Study the drawing (mm; zero at the part's minimum x, y, z) and answer. Coordinates: 2 decimals unless noted, no trailing zeros. Order: outer loops, then holes, each group sorted by start corner. A loop starts at its lowest first (then second) coordinate and runs counter-clockwise, first axis right, second up. Notation, with made-up numbers: (-6, 34) - (14, 34) arc R28 cw to (14, 71) - close; hole circle Ø3 at (49, 63.25). An arc over 180 degrees is marked (long way). Write item = value, one per line.
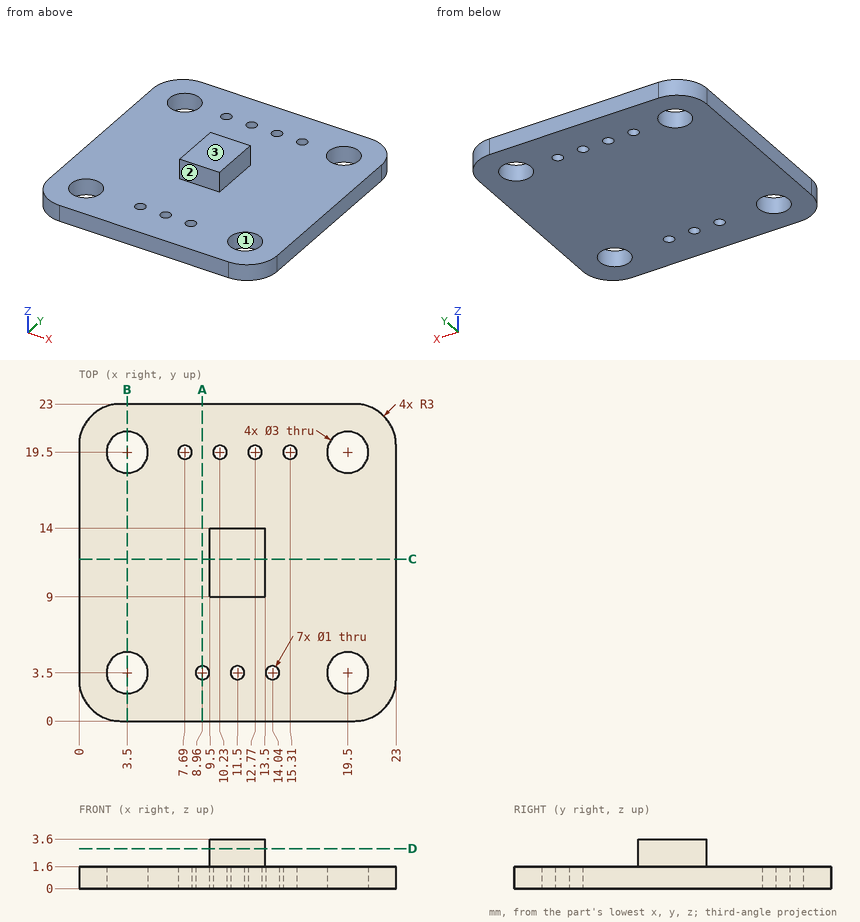
1) Flat-ended cylindrical pins translate along their axes: pin 1 Ø5 at (x, y) = (3.5, 3.5) entering from +Z; pin 2 Ø0.6 at (x, z) = (11, 2.5) entering from +Y; pin 3 Ø2.5 at (x, y) = (3.5, 19.5) entering from -Z; pin 4 Ø2 at (y, z) = (10.5, 3) entering from +X. Find the tip coordinate at first contact, or state that the pin passes through.
Returned:
pin_1 = 1.6
pin_2 = 14
pin_3 = through
pin_4 = 13.5
2) Straight lines are drawn through the part: line 1 along Y through (x, z) = (19.5, 0.9); line 2 along Y through (x, z) = (12.77, 0.6); line 3 along Y through (x, z) = (11.5, 1). For each, find the intervals that lie inside material, in ascending order. Write a range as from..to.
Returned:
line_1 = 0..2, 5..18, 21..23
line_2 = 0..19, 20..23
line_3 = 0..3, 4..23
3) The part is cut by section D-D (z = 2.9). Determine the outline of the cut face in (x, y).
Returned:
outline = (9.5, 9) - (13.5, 9) - (13.5, 14) - (9.5, 14) - close
4) The part is cut by section B-B (x = 3.5). Determine the outline of the cut face in (y, z).
Returned:
outline = (0, 0) - (2, 0) - (2, 1.6) - (0, 1.6) - close; (5, 0) - (18, 0) - (18, 1.6) - (5, 1.6) - close; (21, 0) - (23, 0) - (23, 1.6) - (21, 1.6) - close
5) The part is cut by section A-A (x = 8.96). Determine the outline of the cut face in (y, z).
Returned:
outline = (0, 0) - (3, 0) - (3, 1.6) - (0, 1.6) - close; (4, 0) - (23, 0) - (23, 1.6) - (4, 1.6) - close
6) The part is cut by section C-C (y = 11.75). Determine the outline of the cut face in (x, z).
Returned:
outline = (0, 0) - (23, 0) - (23, 1.6) - (13.5, 1.6) - (13.5, 3.6) - (9.5, 3.6) - (9.5, 1.6) - (0, 1.6) - close
7) Determine the mould class of the marked faces 1, 2 and 3 for opening direction Y: pulls with the +Y half, pulls with the -Y half, needs draft (parallel to the pull), parting line crosses it, or undercut.
Returned:
face_1 = undercut
face_2 = pulls with the -Y half
face_3 = needs draft
